The listing builds one solid part. Answer for the finished solid, in the listing's coordinates (mm). A direction names the side the tool comes from. Coordinates: 2 decimals unless noted, no trailing zeros. Loops run counter-clockwise (first coordinate to the right, second up) from the corner with the lowest first, then second, coordinate; pieces in that order, holes last. Notation, with made-up numbers: M 77.25,31.5 L 122.25,31.5 A25 ccw 122.25,70.5 Z; hole C 20.25,85.5 d11. An arc over 180 degrees is marked long. Return JSON: item names as keys, results as strings. Group by question number.
1. Section B-B (z = -15) is taken. Write down the section's boundary in (x, y), then the cut area to 3 significant figures.
2. Straight lines are drawn through the part: L1, parallel to X at y = 1.55, z = -20; L2, parallel to Z at x = -90, y = 1; L3, parallel to X at y = 0.4, z = 20. For each, find the intervals that lie inside material, in ascending order. Write a range as from..to.
3. Given P1, Ø3, axis at x = -90, z = -20, coming from the +Y side; P2, Ø2.5, axis at x = -90, z = 20, coming from the -Y side; P3, Ø1, axis at x = -38.5, z = 0.5, coming from the -Y side, each flat-ended and moving along its own axis, determine where each tip first touches the part or whether it passes through.
4. Which of the six approach directions +Z, -Z, +X, -X, +Y, -Y give full straight-line access (tool end or side, diameter ignored) to faces 1 (the face through (25.564, -8.162, -2.693)), 2 (the face through (-1, 2, 0))?
5. Section C-C (x = 60) is taken. Write down the section's boundary in (y, z), then the cut area to 3 significant figures.
6. The mould has two halves that part along X. Classify faces 3 (the face through (-38.043, -8.162, -5.651)), 4 (the face through (-93, 1, -34)), 5 (the face through (-43, -14.5, -5)): pulls with the +X half, pulls with the -X half, needs draft (parallel to the pull), parting line crosses it, or undercut.
7. Section A-A (y = -10.25) is taken. Write down the section's boundary in (x, z).
```python
from build123d import *

# Parameters (mm, degrees)
SKETCH_1_R        = 1
SKETCH_1_W        = 5.08
SKETCH_1_H        = 12.7
SKETCH_1_H_2      = 17.78
EXTRUDE_583_DEPTH = 2
SKETCH_2_R        = 5
EXTRUDE_781_DEPTH = 14.5
FILLET_1_SIZE     = 2


with BuildPart() as part:
    # Эскиз1 → Extrude 583 (new body)
    with BuildSketch(Plane(origin=(0, 0, 0), x_dir=(1, 0, 0), z_dir=(0, 1, 0))):
        with BuildLine():
            Line((90, 35), (-90, 35))
            ThreePointArc((-90, 35), (-93.535533906, 33.535533906), (-95, 30))
            Line((-95, 30), (-95, -35))
            Line((-95, -35), (95, -35))
            Line((95, -35), (95, 30))
            ThreePointArc((95, 30), (93.535533906, 33.535533906), (90, 35))
        make_face()
        with Locations(Location((-90, 20, 0), (0, 0, 270))):
            Circle(SKETCH_1_R, mode=Mode.SUBTRACT)
        with Locations(Location((-90, -20, 0), (0, 0, 270))):
            Circle(SKETCH_1_R, mode=Mode.SUBTRACT)
        with Locations(Location((90, -20, 0), (0, 0, 90))):
            Circle(SKETCH_1_R, mode=Mode.SUBTRACT)
        with Locations(Location((90, 20, 0), (0, 0, 90))):
            Circle(SKETCH_1_R, mode=Mode.SUBTRACT)
        with Locations((36.46, -18.65)):
            Rectangle(SKETCH_1_W, SKETCH_1_H, mode=Mode.SUBTRACT)
        with Locations((-25.46, 4.11)):
            Rectangle(SKETCH_1_W, SKETCH_1_H_2, mode=Mode.SUBTRACT)
    extrude(amount=EXTRUDE_583_DEPTH)

    # Эскиз2 → Extrude 781 (add)
    with BuildSketch(Plane(origin=(0, 0, 0), x_dir=(1, 0, 0), z_dir=(0, 1, 0))):
        with Locations(Location((30, 5, 0), (0, 0, 270))):
            Circle(SKETCH_2_R)
        with Locations(Location((-43, 5, 0), (0, 0, 270))):
            Circle(SKETCH_2_R)
    extrude(amount=-EXTRUDE_781_DEPTH)

    # Скругление1
    # a fillet whose section is not a circle: 2 mm, written as the material it adds along each edge
    with BuildSketch(Plane(origin=(30, 0, -5), x_dir=(0, 0, 1), z_dir=(-1, 0, 0))) as fillet_1_piece_1:
        with BuildLine():
            Bezier((5 + FILLET_1_SIZE, 0), (5, 0), (5, -FILLET_1_SIZE), weights=[1, 0.141421356, 1])
            Line((5, -FILLET_1_SIZE), (5, 0))
            Line((5, 0), (5 + FILLET_1_SIZE, 0))
        make_face()
    revolve(axis=Axis((30, 0, -5), (0, 1, 0)))
    with BuildSketch(Plane(origin=(-43, 0, -5), x_dir=(0, 0, 1), z_dir=(-1, 0, 0))) as fillet_1_piece_2:
        with BuildLine():
            Bezier((5 + FILLET_1_SIZE, 0), (5, 0), (5, -FILLET_1_SIZE), weights=[1, 0.141421356, 1])
            Line((5, -FILLET_1_SIZE), (5, 0))
            Line((5, 0), (5 + FILLET_1_SIZE, 0))
        make_face()
    revolve(axis=Axis((-43, 0, -5), (0, 1, 0)))


solid = part.part
```
Worked out:
{
 "1": {"outline": "M -95,0 L 95,0 L 95,2 L -95,2 Z", "area": "380 mm^2"},
 "2": {"L1": "-95..-91, -89..89, 91..95", "L2": "-35..-21, -19..19, 21..35", "L3": "-95..-91, -89..33.92, 39..89, 91..95"},
 "3": {"P1": "y = 2", "P2": "y = 0", "P3": "y = -0.22"},
 "4": {"face 1": "-Y", "face 2": "+Z, -Z, +X, -X, +Y"},
 "5": {"outline": "M 0,-35 L 2,-35 L 2,35 L 0,35 Z", "area": "140 mm^2"},
 "6": {"face 3": "undercut", "face 4": "pulls with the -X half", "face 5": "needs draft"},
 "7": {"outline": "C -43,-5 d10; C 30,-5 d10"}
}
